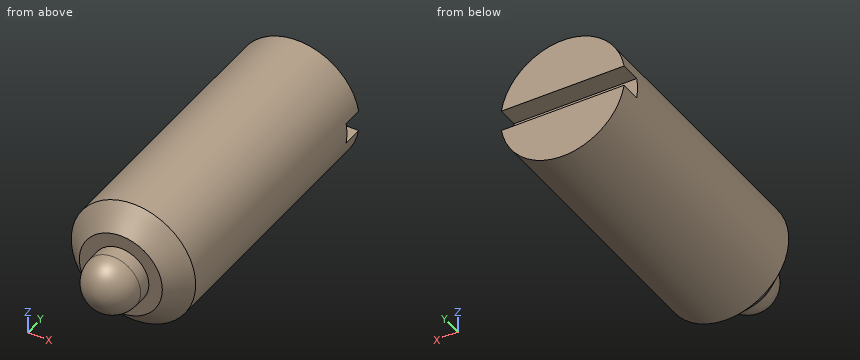
```python
from build123d import *

# Parameters (mm, degrees)
CHAMFER1_SIZE      = 1
SKETCH2_W          = 6.946191838
SKETCH2_H          = 1
CUT_EXTRUDE1_DEPTH = 1


with BuildPart() as part:
    # Sketch1 → Revolve1 (revolve)
    with BuildSketch(Plane.XY, mode=Mode.PRIVATE) as revolve1_sk:
        with BuildLine():
            Line((-1.35, -14), (-1.35, -14.65))
            ThreePointArc((-1.35, -14.65), (-0.954594155, -15.604594155), (0, -16))
            Line((0, -16), (0, 0))
            Line((0, 0), (-3, 0))
            Line((-3, 0), (-3, -14))
            Line((-3, -14), (-1.35, -14))
        make_face()
    revolve(revolve1_sk.sketch.rotate(Axis((0, -16, 0), (0, 1, 0)), 180), axis=Axis((0, -16, 0), (0, 1, 0)))

    # Chamfer1
    chamfer1_edges = [part.edges().sort_by_distance(p)[0] for p in [
        (-3, -14, 0),
    ]]
    chamfer(chamfer1_edges, length=CHAMFER1_SIZE)

    # Sketch2 → Cut-Extrude1 (cut)
    with BuildSketch(Plane(origin=(0, 0, 0), x_dir=(1, 0, 0), z_dir=(0, 1, 0))):
        Rectangle(SKETCH2_W, SKETCH2_H)
    extrude(amount=-CUT_EXTRUDE1_DEPTH, mode=Mode.SUBTRACT)


solid = part.part
```
Could you check a few things on this model? Use its own coordinates, in mm. Round coordinates to 2 decimals unless told otherwise and drop trailing zeros. Loops run counter-clockwise (first coordinate to the right, second up) from the corner with the lowest first, then second, coordinate; pieces in that order, holes last. Notation, with made-up numbers: (28, 32) - (38, 32) arc R7 cw to (38, 39) - close; hole circle Ø8 at (-31, 57.25). An arc over 180 degrees is marked (long way). Answer as CSV lines item,"result".
1. I want a section at D-D on y = -14.5. List the corners of the cut face in (x, z) for me.
Filled in:
outline,"circle Ø2.7 at (0, 0)"
2. Please list where these lines run through material, in increasing order: line 1 along Y through (x, z) = (1.3, -1.5); line 2 along X through (y, z) = (-3.5, 0.15); line 3 along Y through (x, z) = (-1.75, 0.35). Write a range as [from, to].
Filled in:
line 1,"y = [-14, 0]"
line 2,"x = [-3, 3]"
line 3,"y = [-14, -1]"
3. I want a section at C-C on y = -3.25. List the corners of the cut face in (x, z) for me, then the cut area to 3 significant figures.
Filled in:
outline,"circle Ø6 at (0, 0)"
area,"28.3 mm^2"
4. I want a section at B-B on x = 0. List the corners of the cut face in (y, z) for me.
Filled in:
outline,"(-14.65, -1.35) - (-14, -1.35) - (-14, -2) - (-13, -3) - (0, -3) - (0, -0.5) - (-1, -0.5) - (-1, 0.5) - (0, 0.5) - (0, 3) - (-13, 3) - (-14, 2) - (-14, 1.35) - (-14.65, 1.35) arc R1.35 ccw to start"
5. I want a section at A-A on z = 0. List the corners of the cut face in (x, y) for me, then the cut area to 3 significant figures.
Filled in:
outline,"(-3, -13) - (-2, -14) - (-1.35, -14) - (-1.35, -14.65) arc R1.35 ccw to (1.35, -14.65) - (1.35, -14) - (2, -14) - (3, -13) - (3, -1) - (-3, -1) - close"
area,"81.6 mm^2"
6. For pin 1 Ø0.8 at (x, z) = (-1, 0) entering from +Y; pin 2 Ø2 at (x, y) = (2, -6) entering from +Z; pin 3 Ø1.5 at (x, y) = (2, -7.5) entering from +Z, each with a flat end and sliding along its axis, tell me the tip position at first contact or that it passes through.
Filled in:
pin 1,"stops at y = -1"
pin 2,"stops at z = 2.83"
pin 3,"stops at z = 2.73"
